Input: part model. Units: mm. Frame: model coordinates. Face numbers are marked on the shaded views. A direction names the side the tool comes from. Give positions to 0.01 mm unless a question says otherwise; leave off trailing zeros. Loops run counter-clockwise (first coordinate to the right, second up) from the corner with the lowest first, then second, coordinate; pieces in that order, holes last. Notation, with made-up numbers: (5.25, 78) - (22.25, 78) arc R27 ccw to (22.25, 100) - close; hole circle Ø3 at (-8, 29.5). An arc over 180 degrees is marked (long way). Answer as a JSON object with one key per item and string values.
from build123d import *

# Parameters (mm, degrees)
ESQUISSE1_W             = 40
ESQUISSE1_H             = 40
BOSS_EXTRU_1_DEPTH      = 25
ESQUISSE2_R             = 4
ENL_V_MAT_EXTRU_1_DEPTH = 47
ESQUISSE4_R             = 4
BOSS_EXTRU_3_DEPTH      = 5


with BuildPart() as part:
    # Esquisse1 → Boss.-Extru.1 (new body)
    with BuildSketch(Plane.XY):
        Rectangle(ESQUISSE1_W, ESQUISSE1_H)
    extrude(amount=BOSS_EXTRU_1_DEPTH)

    # Esquisse2 → Enlèv. mat.-Extru.1 (cut)
    with BuildSketch(Plane(origin=(0, 20, 0), x_dir=(1, 0, 0), z_dir=(0, 1, 0))):
        with Locations((7.492941833, -12.5)):
            Circle(ESQUISSE2_R)
    extrude(amount=-ENL_V_MAT_EXTRU_1_DEPTH, mode=Mode.SUBTRACT)

    # Esquisse4 → Boss.-Extru.3 (add)
    with BuildSketch(Plane(origin=(0, 20, 0), x_dir=(1, 0, 0), z_dir=(0, 1, 0))):
        with BuildLine():
            Line((-20, -25), (-34.7092612, -22.061014641))
            ThreePointArc((-34.7092612, -22.061014641), (-42.749937628, -12.254840508), (-34.7092612, -2.448666374))
            Line((-34.7092612, -2.448666374), (-20, 0))
            Line((-20, 0), (-20, -25))
        make_face()
        with Locations((-32.749937628, -12.254840508)):
            Circle(ESQUISSE4_R, mode=Mode.SUBTRACT)
    boss_extru_3 = extrude(amount=-BOSS_EXTRU_3_DEPTH)

    # Symétrie2: Boss.-Extru.3 across plane
    add(boss_extru_3.mirror(Plane.ZX))


solid = part.part
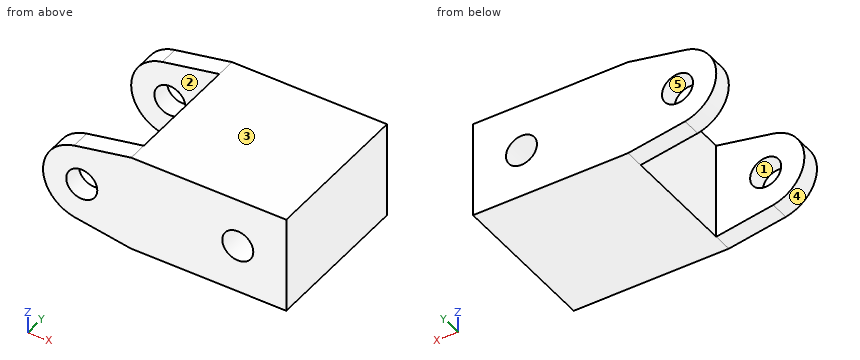
Item 1: Mould query, pull axis X, two halves, no side actions, for the marked faces 3, 4 and 5. Classes: released by +X, released by -X, zero draft, split by the parting line, or undercut.
Geometry check:
{"face 3": "zero draft", "face 4": "released by -X", "face 5": "undercut"}
Item 2: Contact query for flat-ended pins moving along their axis: P1, Ø5, axis at x = -32.75, z = 12.25, coming from the -Y side; P2, Ø12.5, axis at y = 2, z = 10.5, coming from the -X side. Output: stop coordinate, or through.
Geometry check:
{"P1": "passes through", "P2": "stops at x = -20"}
Item 3: Cut plane A-A (z = 15.5). Return loops of the section in (x, y).
Geometry check:
{"outline": "(-42.21, -20) - (-35.09, -20) - (-35.09, -15) - (-42.21, -15) - close; (-42.21, 15) - (-35.09, 15) - (-35.09, 20) - (-42.21, 20) - close; (-30.41, -20) - (4.85, -20) - (4.85, 20) - (-30.41, 20) - (-30.41, 15) - (-20, 15) - (-20, -15) - (-30.41, -15) - close; (10.14, -20) - (20, -20) - (20, 20) - (10.14, 20) - close"}
Item 4: Material intervals for line 1 (Y direction, x = -38, z = 13); line 2 (X direction, y = 11, z = 12.5); line 3 (X direction, y = -15.5, z = 11.5), sorted ascending. Write a range as [from, to].
Geometry check:
{"line 1": "y = [-20, -15], [15, 20]", "line 2": "x = [-20, 3.49], [11.49, 20]", "line 3": "x = [-42.72, -36.68], [-28.82, 3.62], [11.37, 20]"}
Item 5: Access query for the marked faces 1 and 2. Directions: +Z, -Z, +X, -X, +Y, -Y. A direction counts if a zero-diameter tool reaches every point of the face in a straight line with its end or side. Return the directions, or none.
Geometry check:
{"face 1": "+Y, -Y", "face 2": "+Z, -Z, -X"}
Item 6: Cut plane B-B (y = -1). Return loops of the section in (x, z), then the cut area to 3 significant figures.
Geometry check:
{"outline": "(-20, 0) - (20, 0) - (20, 25) - (-20, 25) - close; hole circle Ø8 at (7.49, 12.5)", "area": "950 mm2"}
Item 7: Cut plane C-C (z = 5). Return loops of the section in (x, y), then the cut area to 3 significant figures.
Geometry check:
{"outline": "(-39.63, -20) - (20, -20) - (20, 20) - (-39.63, 20) - (-39.63, 15) - (-20, 15) - (-20, -15) - (-39.63, -15) - close", "area": "1,800 mm2"}
